```python
from build123d import *

# Parameters (mm, degrees)
F0_R     = 2
F1_DEPTH = 10
F2_W     = 8
F2_H     = 8
F2_R     = 2
F3_DEPTH = 10


with BuildPart() as f1:
    # F0 (on Right) → F1 (new body)
    with BuildSketch(Plane.YZ):
        Polygon((2.5, -4), (2.5, 4), (-2.5, 4), (-2.5, 20), (13.5, 20), (13.5, 28), (-10.5, 28), (-10.5, -12), (-2.5, -12), (-2.5, -4), align=None)
        with Locations((9.5, 24)):
            Circle(F0_R, mode=Mode.SUBTRACT)
    extrude(amount=F1_DEPTH)

    # F2 (on face) → F3 (join)
    with BuildSketch(Plane(origin=(0, 0, 0), x_dir=(0, -1, 0), z_dir=(-1, 0, 0))):
        Polygon((-13.5, -2), (-13.5, 20), (-13.5, 28), (-21.5, 28), (-21.5, -2), align=None)
        with Locations((-9.5, 24)):
            Rectangle(F2_W, F2_H)
        with Locations((-9.5, 24)):
            Circle(F2_R, mode=Mode.SUBTRACT)
    extrude(amount=F3_DEPTH)


solid = f1.part
```
Check sheet for the modelled part. Datum: model origin and axes. Units: mm. A direction names the side the tool comes from. Give positions to 0.01 mm unless a question says otherwise; leave off trailing zeros. Loops run counter-clockwise (first coordinate to the right, second up) from the corner with the lowest first, then second, coordinate; pieces in that order, holes last. Notation, with made-up numbers: (72, 53.5) - (81, 53.5) arc R34 ccw to (81, 90.5) - close; hole circle Ø11 at (74.25, -11). An arc over 180 degrees is marked (long way). One line per question, with ' | ' between items. Start each with the question number.
1. Cross-section at A-A, the plane z = 2.5. Enter the section's corners in (x, y), plus the area to 3 significant figures.
2. Cross-section at D-D, the plane z = 24. Enter the section's corners in (x, y), plus the area to 3 significant figures.
3. Draft check along Z on faces 4 (the flat face through (5, 0, 4)), 5 (the flat face through (0, -4, 8)), 6 (the flat face through (-5, 18, -2)). Enter one of: released by +Z, released by -Z, zero draft, split by the parting line, or undercut.
4. Cross-section at C-C, the plane y = 9.5. Enter the section's corners in (x, z).
5. Material ranges on line 1 along Z through (x, y) = (3.5, 9.5); line 2 along Y through (x, z) = (-3.5, 24); line 3 along Y through (x, z) = (4, 24), recorded low to high. Write a range as [from, to].
6. Set-up check for faces 1 (the flat face through (-5, 5.5, 24)), 2 (the flat face through (5, -2.5, -8)), 3 (the flat face through (0, 18, 13)): record each of +Z, -Z, +X, -X, +Y, -Y from which the full face is reachable in a straight line by a thin tool's end or side.
7. Cross-section at B-B, the plane x = -6.5. Enter the section's corners in (y, z), plus the area to 3 significant figures.
8. Gauge pin test, flat ends, axial feed: pin 1 Ø4 at (x, z) = (6.5, 0.5) entering from +Y; pin 2 Ø12 at (y, z) = (6, 8.5) entering from -X; pin 3 Ø5 at (x, y) = (0, 3.5) entering from -Z; pin 4 Ø6 at (x, z) = (2.5, 1.5) entering from +Y. Record the tip position at first contact, or that the pin passes through.
Check result:
1) outline: (-10, 13.5) - (0, 13.5) - (0, 21.5) - (-10, 21.5) - close; (0, -10.5) - (10, -10.5) - (10, 2.5) - (0, 2.5) - close | area: 210 mm2
2) outline: (-10, 5.5) - (0, 5.5) - (0, -10.5) - (10, -10.5) - (10, 7.5) - (-10, 7.5) - close; (-10, 11.5) - (10, 11.5) - (10, 13.5) - (0, 13.5) - (0, 21.5) - (-10, 21.5) - close | area: 320 mm2
3) face 4: undercut | face 5: zero draft | face 6: released by -Z
4) outline: (-10, 20) - (10, 20) - (10, 22) - (-10, 22) - close; (-10, 26) - (10, 26) - (10, 28) - (-10, 28) - close
5) line 1: z = [20, 22], [26, 28] | line 2: y = [5.5, 7.5], [11.5, 21.5] | line 3: y = [-10.5, 7.5], [11.5, 13.5]
6) face 1: +Z, -Z, -X, -Y | face 2: -Z, +X, -X, +Y | face 3: +Z, -Z, +X, +Y
7) outline: (5.5, 20) - (13.5, 20) - (13.5, -2) - (21.5, -2) - (21.5, 28) - (5.5, 28) - close; hole circle Ø4 at (9.5, 24) | area: 291 mm2
8) pin 1: stops at y = 2.5 | pin 2: stops at x = 0 | pin 3: stops at z = -4 | pin 4: stops at y = 21.5
